Source: CAD feature listing. Evaluate the final solid. Frame: model axes, mm. Face numbers are marked on the shaded views. A direction names the side the tool comes from. Give positions to 0.01 mm unless a question says otherwise; leave off trailing zeros. Write each loop counter-clockwise with the first axis right and the second up, starting at its lowest first coordinate (ties: lowest second). Pieces come first, ordered by that corner, then holes. Notation, with made-up numbers: (83.5, 67.25) -> (138.5, 67.25) arc R23 ccw to (138.5, 104.25) -> close; hole circle Ø2 at (61.25, 43.25). An arc over 180 degrees is marked (long way). Answer as a JSON object with one key per item and string values. Group by question number.
Item 1: Section query D-D on z = -10.5. Return the cut outline in (x, y), plus the area to 3 significant figures.
Item 2: Ray query, probe 1 along X at (y, z) = (6, 0); probe 2 along Y at (x, z) = (4, 4.75); probe 3 along Y at (x, z) = (-8.5, -9). Return the intervals inside material, ascending. Write a range as from..to.
Item 3: Section query C-C on y = 6. Return the cut outline in (x, z), plus the area to 3 significant figures.
Item 4: First-contact query: pin 1 Ø12 at (x, y) = (-8, 20.5) entering from +Z; pin 2 Ø2 at (x, z) = (-4.5, -10.5) entering from -Y; pin 3 Ø1.5 at (y, z) = (16.5, 10.5) entering from -X; pin 4 Ø6 at (x, y) = (-6, 12) entering from +Z. Flat tips, straight axial feed; report the tip coordinate or a pass-through.
Item 5: Section query A-A on x = 0. Return the cut outline in (y, z).
Item 6: Pull-direction query (Y, two-part tool) for the marked faces 1, 2, 3 and 4; classes: pulls with the +Y half, pulls with the -Y half, needs draft (parallel to the pull), parting line crosses it, or undercut.
Item 7: Section query B-B on z = 0. Return the cut outline in (x, y), plus the area to 3 significant figures.
Item 8: Access query for the marked faces 5 and 6. Directions: +Z, -Z, +X, -X, +Y, -Y. A direction counts if a zero-diameter tool reaches every point of the face in a straight line with its end or side. Return the directions, or none.
from build123d import *

# Parameters (mm, degrees)
SKETCH1_R               = 15
BOSS_EXTRUDE1_DEPTH     = 25
SKETCH2_R               = 3
CUT_EXTRUDE1_DEPTH      = 25
SKETCH3_W               = 0.8
SKETCH3_H               = 3.945833246
BOSS_EXTRUDE2_DEPTH     = 25
CUT_EXTRUDE2_DEPTH      = 2000
CUT_EXTRUDE2_DEPTH_BACK = 25
SKETCH4_R               = 1.25
SKETCH5_W               = 6
SKETCH5_H               = 21


with BuildPart() as part:
    # Sketch1 → Boss-Extrude1 (new body)
    with BuildSketch(Plane(origin=(0, 0, 0), x_dir=(1, 0, 0), z_dir=(0, 1, 0))):
        with Locations(Location((0, 0, 0), (0, 0, 270))):
            Circle(SKETCH1_R)
    extrude(amount=BOSS_EXTRUDE1_DEPTH)

    # Sketch2 → Cut-Extrude1 (cut)
    with BuildSketch(Plane(origin=(0, 25, 0), x_dir=(1, 0, 0), z_dir=(0, 1, 0))):
        with Locations(Location((0, 0, 0), (0, 0, 270))):
            Circle(SKETCH2_R)
    extrude(amount=-CUT_EXTRUDE1_DEPTH, mode=Mode.SUBTRACT)

    # Sketch3 → Boss-Extrude2 (add)
    with BuildSketch(Plane(origin=(0, 0, 0), x_dir=(1, 0, 0), z_dir=(0, 1, 0))):
        with Locations((2.66, 0)):
            Rectangle(SKETCH3_W, SKETCH3_H)
    extrude(amount=BOSS_EXTRUDE2_DEPTH)

    # Sketch4 → Cut-Extrude2 (cut, two sides: drawn at the far end of the back side and taken through both)
    with BuildSketch(Plane.XY.offset(-CUT_EXTRUDE2_DEPTH_BACK)):
        with Locations(Location((4, 6, 0), (0, 0, 180))):
            Circle(SKETCH4_R)
    extrude(amount=CUT_EXTRUDE2_DEPTH + CUT_EXTRUDE2_DEPTH_BACK, mode=Mode.SUBTRACT)

    # Sketch5 → Cut-Revolve1 (revolve, cut)
    with BuildSketch(Plane.XY, mode=Mode.PRIVATE) as cut_revolve1_sk:
        with Locations((12, 12.5)):
            Rectangle(SKETCH5_W, SKETCH5_H)
    revolve(cut_revolve1_sk.sketch.rotate(Axis((0, 0, 0), (0, 1, 0)), 90), axis=Axis((0, 0, 0), (0, 1, 0)), mode=Mode.SUBTRACT)


solid = part.part
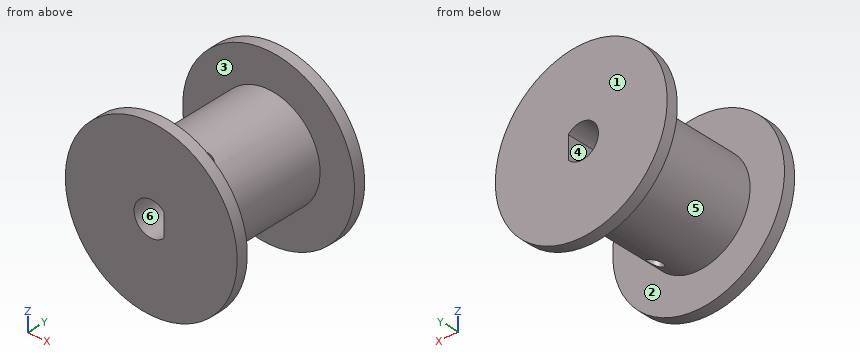
Worked answers:
{
 "1": {"outline": "(-10.71, 0) -> (10.71, 0) -> (10.71, 2) -> (-10.71, 2) -> close; (-10.71, 23) -> (10.71, 23) -> (10.71, 25) -> (-10.71, 25) -> close", "area": "85.7 mm^2"},
 "2": {"probe 1": "-9..-3, 2.26..2.75, 5.25..9", "probe 2": "0..4.75, 7.25..25", "probe 3": "0..2, 23..25"},
 "3": {"outline": "(2.75, -8.57) -> (2.75, 8.57) arc R9 ccw (long way) to start; (5.25, -7.31) arc R9 ccw to (5.25, 7.31) -> close; hole (2.26, -1.97) -> (2.26, 1.97) arc R3 ccw (long way) to start", "area": "188 mm^2"},
 "4": {"pin 1": "z = 14.78", "pin 2": "y = 0", "pin 3": "through", "pin 4": "z = 8.49"},
 "5": {"outline": "(0, -15) -> (2, -15) -> (2, -9) -> (23, -9) -> (23, -15) -> (25, -15) -> (25, -3) -> (0, -3) -> close; (0, 3) -> (25, 3) -> (25, 15) -> (23, 15) -> (23, 9) -> (2, 9) -> (2, 15) -> (0, 15) -> close"},
 "6": {"face 1": "pulls with the +Y half", "face 2": "undercut", "face 3": "undercut", "face 4": "needs draft"},
 "7": {"outline": "(-15, 0) -> (-3, 0) -> (-3, 25) -> (-15, 25) -> (-15, 23) -> (-9, 23) -> (-9, 2) -> (-15, 2) -> close; (2.26, 0) -> (15, 0) -> (15, 2) -> (9, 2) -> (9, 23) -> (15, 23) -> (15, 25) -> (2.26, 25) -> close; hole circle Ø2.5 at (4, 6)", "area": "362 mm^2"},
 "8": {"face 5": "none", "face 6": "+Y, -Y"}
}
